Input: part model. Units: mm. Frame: model coordinates. A direction names the side the tool comes from. Coordinates: 2 decimals unless noted, no trailing zeros. Order: outer loops, then holes, each group sorted by start corner. A loop starts at its lowest first (then second) coordinate and runs counter-clockwise, first axis right, second up. Notation, with made-up numbers: (84.5, -37) -> (114.5, -37) arc R16 cw to (114.5, -7) -> close; hole circle Ø8 at (1, 71.5). An arc over 180 degrees is marked (long way). One line per question, with ' | ' between items.
```python
from build123d import *

# Parameters (mm, degrees)
F0_R     = 6.35
F1_DEPTH = 46.99328
F3_DEPTH = 12.7
F5_D     = 5.08
F5_DEPTH = 25.4
F5_TIP   = 1.5261859723


with BuildPart() as f1:
    # F0 (on Right) → F1 (new body)
    with BuildSketch(Plane.YZ):
        with Locations((42.2567352653, 52.6904910803)):
            Circle(F0_R)
    extrude(amount=F1_DEPTH)

    # F2 (on face) → F3 (join)
    with BuildSketch(Plane(origin=(0, 0, 0), x_dir=(0, -1, 0), z_dir=(-1, 0, 0))):
        with BuildLine():
            Line((-42.2567352653, 59.0404910803), (-48.6067352653, 59.0404910803))
            Line((-48.6067352653, 59.0404910803), (-48.6067352653, 52.6904910803))
            ThreePointArc((-48.6067352653, 52.6904910803), (-46.7468633258, 57.1806191408), (-42.2567352653, 59.0404910803))
        make_face()
        with BuildLine():
            Line((-35.9067352653, 59.0404910803), (-42.2567352653, 59.0404910803))
            ThreePointArc((-42.2567352653, 59.0404910803), (-37.7666072047, 57.1806191408), (-35.9067352653, 52.6904910803))
            Line((-35.9067352653, 52.6904910803), (-35.9067352653, 59.0404910803))
        make_face()
        with BuildLine():
            ThreePointArc((-35.9067352653, 52.6904910803), (-37.7666072047, 57.1806191408), (-42.2567352653, 59.0404910803))
            ThreePointArc((-42.2567352653, 59.0404910803), (-46.7468633258, 57.1806191408), (-48.6067352653, 52.6904910803))
            ThreePointArc((-48.6067352653, 52.6904910803), (-46.7468633258, 48.2003630197), (-42.2567352653, 46.3404910803))
            ThreePointArc((-42.2567352653, 46.3404910803), (-37.7666072047, 48.2003630197), (-35.9067352653, 52.6904910803))
        make_face()
        with BuildLine():
            ThreePointArc((-42.2567352653, 46.3404910803), (-46.7468633258, 48.2003630197), (-48.6067352653, 52.6904910803))
            Line((-48.6067352653, 52.6904910803), (-48.6067352653, 46.3404910803))
            Line((-48.6067352653, 46.3404910803), (-42.2567352653, 46.3404910803))
        make_face()
        with BuildLine():
            Line((-35.9067352653, 46.3404910803), (-35.9067352653, 52.6904910803))
            ThreePointArc((-35.9067352653, 52.6904910803), (-37.7666072047, 48.2003630197), (-42.2567352653, 46.3404910803))
            Line((-42.2567352653, 46.3404910803), (-35.9067352653, 46.3404910803))
        make_face()
    extrude(amount=F3_DEPTH)

    # F5
    with Locations(Plane(origin=(0, 48.6067352653, 0), x_dir=(-1, 0, 0), z_dir=(0, 1, 0))):
        with Locations((6.35, 55.8654910803), (6.35, 49.5154910803)):
            Hole(F5_D / 2, depth=F5_DEPTH)
            with Locations((0, 0, -(F5_DEPTH + F5_TIP / 2))):  # 118° drill point
                Cone(0, F5_D / 2, F5_TIP, mode=Mode.SUBTRACT)


solid = f1.part
```
1. Cut plane B-B, the plane y = 44.75. Return loops of the section in (x, z), and give its area (3 significant figures).
Recorded:
outline: (-12.7, 46.34) -> (0, 46.34) -> (0, 46.85) -> (46.99, 46.85) -> (46.99, 58.53) -> (0, 58.53) -> (0, 59.04) -> (-12.7, 59.04) -> close; hole circle Ø5.08 at (-6.35, 49.52); hole circle Ø5.08 at (-6.35, 55.87) | area: 670 mm^2
2. Pin query (flat end, axial travel): pin 1 Ø1 at (x, z) = (17.5, 51.5) entering from -Y; pin 2 Ø1.5 at (x, z) = (14, 48) entering from +Y; pin 3 Ø5 at (x, y) = (26, 46.5) entering from -Z. Return the tip coordinate at first contact, or that it passes through.
Recorded:
pin 1: stops at y = 35.94 | pin 2: stops at y = 47.24 | pin 3: stops at z = 46.58
3. Mould query, pull axis Z, two halves, no side actions, for faces 1 (the face through (-8.222, 42.168, 57.582)), 2 (the face through (-6, 42, 46.34)), 3 (the face through (-6, 48.607, 53)). Classes: released by +Z, released by -Z, zero draft, split by the parting line, or undercut.
Recorded:
face 1: undercut | face 2: released by -Z | face 3: zero draft
4. Cut plane A-A, the plane x = -6.35. Return loops of the section in (y, z).
Recorded:
outline: (35.91, 46.34) -> (48.61, 46.34) -> (48.61, 46.98) -> (35.91, 46.98) -> close; (35.91, 52.06) -> (48.61, 52.06) -> (48.61, 53.33) -> (35.91, 53.33) -> close; (35.91, 58.41) -> (48.61, 58.41) -> (48.61, 59.04) -> (35.91, 59.04) -> close
5. Ray query, line 1 (Z direction, x = -6.35, y = 40.25); line 2 (X direction, y = 43, z = 49.5); line 3 (X direction, y = 46.5, z = 54.5). Return the intervals inside material, ascending. Write a range as [from, to].
Recorded:
line 1: z = [46.34, 46.98], [52.06, 53.33], [58.41, 59.04] | line 2: x = [-12.7, -8.89], [-3.81, 46.99] | line 3: x = [-12.7, -8.49], [-4.21, 46.99]
6. Cut plane C-C, the plane x = 17. Return loops of the section in (y, z), and give its area (3 significant figures).
Recorded:
outline: circle Ø12.7 at (42.26, 52.69) | area: 127 mm^2
7. Access query for faces 4 (the face through (23.168, 37.218, 48.827)), 5 (the face through (0, 37, 48)), 6 (the face through (0, 37, 58)), 7 (the face through (0, 47, 48)). Directions: +Z, -Z, +X, -X, +Y, -Y. A direction counts if a zero-diameter tool reaches every point of the face in a straight line with its end or side. Return the directions, or none.
Recorded:
face 4: +X | face 5: -Z, +X, -Y | face 6: +Z, +X, -Y | face 7: -Z, +X, +Y
8. Cut plane D-D, the plane y = 38.5. Return loops of the section in (x, z), and give its area (3 significant figures).
Recorded:
outline: (-12.7, 46.34) -> (0, 46.34) -> (0, 47.57) -> (46.99, 47.57) -> (46.99, 57.81) -> (0, 57.81) -> (0, 59.04) -> (-12.7, 59.04) -> close; hole circle Ø5.08 at (-6.35, 49.52); hole circle Ø5.08 at (-6.35, 55.87) | area: 602 mm^2
